Work out the finished part from the listing and answer in its coordinate system (mm). A direction names the side the tool comes from. Coordinates: 2 decimals unless noted, no trailing zeros. Loops run counter-clockwise (first coordinate to the right, second up) from the corner with the lowest first, then second, coordinate; pieces in that order, holes last. Notation, with made-up numbers: (53, 38.5) -> (83, 38.5) arc R6 ccw to (83, 49.5) -> close; hole circle Ø10 at (73.5, 11). An arc over 180 degrees is marked (long way). Use a Markdown table: item, result.
from build123d import *

# Parameters (mm, degrees)
SKETCH1_W           = 60
SKETCH1_H           = 20
BOSS_EXTRUDE1_DEPTH = 5
SKETCH2_W           = 60
SKETCH2_H           = 10
BOSS_EXTRUDE2_DEPTH = 80
SKETCH3_R           = 7.5
CUT_EXTRUDE1_DEPTH  = 5
FILLET1_R           = 10
SKETCH4_R           = 2
CUT_EXTRUDE2_DEPTH  = 92.378334412


with BuildPart() as part:
    # Sketch1 → Boss-Extrude1 (new body)
    with BuildSketch(Plane(origin=(0, 0, 0), x_dir=(1, 0, 0), z_dir=(0, 1, 0))):
        Rectangle(SKETCH1_W, SKETCH1_H)
        with BuildLine():
            Line((-16.8, 8.4), (-5, 8.4))
            ThreePointArc((-5, 8.4), (-1.6, 5), (-5, 1.6))
            Line((-5, 1.6), (-16.8, 1.6))
            ThreePointArc((-16.8, 1.6), (-20.2, 5), (-16.8, 8.4))
        make_face(mode=Mode.SUBTRACT)
        with BuildLine():
            Line((3.2, 8.4), (15, 8.4))
            ThreePointArc((15, 8.4), (18.4, 5), (15, 1.6))
            Line((15, 1.6), (3.2, 1.6))
            ThreePointArc((3.2, 1.6), (-0.2, 5), (3.2, 8.4))
        make_face(mode=Mode.SUBTRACT)
    extrude(amount=BOSS_EXTRUDE1_DEPTH)

    # Sketch2 → Boss-Extrude2 (add)
    with BuildSketch(Plane(origin=(0, 5, 0), x_dir=(1, 0, 0), z_dir=(0, 1, 0))):
        with Locations((0, -5)):
            Rectangle(SKETCH2_W, SKETCH2_H)
    extrude(amount=BOSS_EXTRUDE2_DEPTH)

    # Sketch3 → Cut-Extrude1 (cut)
    with BuildSketch(Plane(origin=(0, 0, 0), x_dir=(-1, 0, 0), z_dir=(0, 0, -1))):
        with Locations((0, 58)):
            Circle(SKETCH3_R)
    extrude(amount=-CUT_EXTRUDE1_DEPTH, mode=Mode.SUBTRACT)

    # Fillet1
    fillet1_edges = [part.edges().sort_by_distance(p)[0] for p in [
        (30, 85, 5),
        (-30, 85, 5),
    ]]
    fillet(fillet1_edges, radius=FILLET1_R)

    # Sketch4 → Cut-Extrude2 (cut, through all)
    with BuildSketch(Plane(origin=(0, 0, 5), x_dir=(-1, 0, 0), z_dir=(0, 0, -1))):
        with Locations((0, 58)):
            Circle(SKETCH4_R)
    extrude(amount=-CUT_EXTRUDE2_DEPTH, mode=Mode.SUBTRACT)


solid = part.part
Q1. Determine the mould class of faces 4 (the flat face through (9, 2, -1.6)), 5 (the flat face through (-30, 37, 5)), 6 (the flat face through (0, 85, 5)) for opening direction X: pulls with the +X half, pulls with the -X half, needs draft (parallel to the pull), parting line crosses it, or undercut.
Solved:
| item | result |
|---|---|
| face 4 | undercut |
| face 5 | pulls with the -X half |
| face 6 | needs draft |
Q2. Given pin 1 Ø13.5 at (x, y) = (0, 58) entering from -Z; pin 2 Ø7.5 at (x, y) = (-2.5, 55) entering from -Z; pin 3 Ø8 at (x, z) = (0, -5) entering from +Y; pin 4 Ø3 at (x, y) = (0, 58) entering from +Z, each flat-ended and moving along its own axis, determine where each tip first touches the part or whether it passes through.
Solved:
| item | result |
|---|---|
| pin 1 | z = 5 |
| pin 2 | z = 0 |
| pin 3 | y = 5 |
| pin 4 | through |
Q3. Section A-A on x = -15.5 is taken. Determine the outline of the cut face in (y, z).
Solved:
| item | result |
|---|---|
| outline | (0, -10) -> (5, -10) -> (5, -8.4) -> (0, -8.4) -> close; (0, -1.6) -> (5, -1.6) -> (5, 0) -> (85, 0) -> (85, 10) -> (0, 10) -> close |
Q4. Section B-B on y = 58 is taken. Determine the outline of the cut face in (x, z).
Solved:
| item | result |
|---|---|
| outline | (-30, 0) -> (-7.5, 0) -> (-7.5, 5) -> (-2, 5) -> (-2, 10) -> (-30, 10) -> close; (2, 5) -> (7.5, 5) -> (7.5, 0) -> (30, 0) -> (30, 10) -> (2, 10) -> close |
Q5. Section D-D on y = 67.5 is taken. Determine the outline of the cut face in (x, z), and give its area (3 significant figures).
Solved:
| item | result |
|---|---|
| outline | (-30, 0) -> (30, 0) -> (30, 10) -> (-30, 10) -> close |
| area | 600 mm² |
Q6. Consider line 1 (Y direction, x = 0, z = 7.35); line 2 (Z direction, x = -20, y = 29); line 3 (Y direction, x = 0, z = 1.2). Determine where each line is inside the solid, lowest interval first. Write a range as [from, to].
Solved:
| item | result |
|---|---|
| line 1 | [0, 56], [60, 85] |
| line 2 | [0, 10] |
| line 3 | [0, 50.5], [65.5, 85] |
Q7. Section C-C on z = -5 is taken. Determine the outline of the cut face in (x, y).
Solved:
| item | result |
|---|---|
| outline | (-30, 0) -> (-20.2, 0) -> (-20.2, 5) -> (-30, 5) -> close; (-1.6, 0) -> (-0.2, 0) -> (-0.2, 5) -> (-1.6, 5) -> close; (18.4, 0) -> (30, 0) -> (30, 5) -> (18.4, 5) -> close |
Q8. For faces 1 (the cylindrical face through (-20.2, 2.5, -4.9)), 2 (the cylindrical face through (0.976, 65.436, 2.465)), 3 (the flat face through (-0.4, 5, -5.1)), determine the directions among +Z, -Z, +X, -X, +Y, -Y from which every point of the face is accessible in a straight line to the end or side of a thin tool.
Solved:
| item | result |
|---|---|
| face 1 | +Y, -Y |
| face 2 | -Z |
| face 3 | -Z, +X, -X, +Y |
